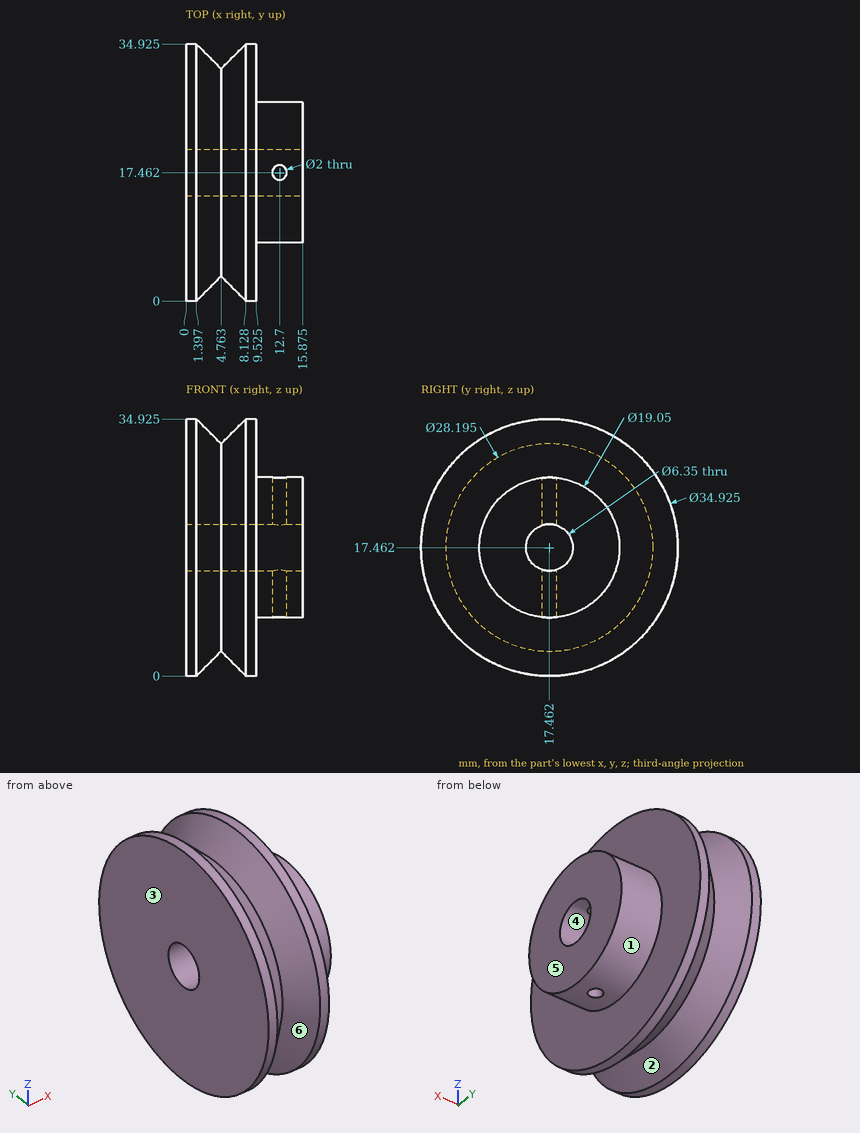
Geometry check sheet. Reference: drawing and pictorial views, mm from the part's lowest x, y, z. A direction names the side the tool comes from. Round coordinates to 2 decimals unless told otherwise and drop trailing zeros. Use a Markdown table: item, result. Add a question column.
1. Gauge pin test, flat ends, axial feed: pin 1 (1.5 mm diameter, centred on x = 8, y = 21.5, fed in from -Z) (1 decimal); pin 2 (1.8 mm diameter, centred on x = 12.7, y = 17.46, fed in from -Z); pin 3 (1 mm diameter, centred on x = 11, z = 16.5, fed in from -Y); pin 4 (4 mm diameter, centred on x = 1.5, z = 20, fed in from -Y). Record the tip position at first contact, or that the pin passes through.
2. Release check for a two-part mould opening along Y. For the marked faces 4, 5 and 6 record: released by +Y, released by -Y, zero draft, split by the parting line, or undercut.
3. Thickness scan on probe 1 along Z at (x, y) = (8.5, 17.5) (1 decimal); probe 2 along X at (y, z) = (26, 23) (1 decimal); probe 3 along Z at (x, y) = (1, 18.5) (1 decimal). Record the ranges inside material, lowest first. Write a range as [from, to].
4. Access from +Z, -Z, +X, -X, +Y, -Y to the whole of each face (thin tool, end or side, straight path). Record for the marked faces 1, 2 and 3.
Checks:
| question | item | result |
|---|---|---|
| 1 | pin 1 | stops at z = 0.3 |
| 1 | pin 2 | passes through |
| 1 | pin 3 | stops at y = 7.95 |
| 1 | pin 4 | stops at y = 0.01 |
| 2 | face 4 | undercut |
| 2 | face 5 | zero draft |
| 2 | face 6 | split by the parting line |
| 3 | probe 1 | z = [0, 14.3], [20.6, 34.9] |
| 3 | probe 2 | x = [0, 9.5] |
| 3 | probe 3 | z = [0, 14.5], [20.5, 34.9] |
| 4 | face 1 | +X |
| 4 | face 2 | none |
| 4 | face 3 | +Z, -Z, -X, +Y, -Y |
